from build123d import *

# Parameters (mm, degrees)
SKETCH_2_R          = 21
SKETCH_2_R_2        = 2.5
EXTRUDE_1_DEPTH     = 3
FILLET_1_R          = 1.5
SKETCH_3_R          = 1.45
CUT_EXTRUDE_1_DEPTH = 5
FILLET_2_R          = 3


with BuildPart() as part:
    # Sketch 2 → Extrude 1 (new body)
    with BuildSketch(Plane.XY):
        with BuildLine():
            Line((-10, -58), (10, -58))
            Line((10, -58), (27.296195268, -9.793759437))
            ThreePointArc((27.296195268, -9.793759437), (0, 29), (-27.296195268, -9.793759437))
            Line((-27.296195268, -9.793759437), (-10, -58))
        make_face()
        Circle(SKETCH_2_R, mode=Mode.SUBTRACT)
        with Locations((0, 24.5)):
            Circle(SKETCH_2_R_2, mode=Mode.SUBTRACT)
        with Locations((21.217622393, 12.25)):
            Circle(SKETCH_2_R_2, mode=Mode.SUBTRACT)
        with Locations((21.217622393, -12.25)):
            Circle(SKETCH_2_R_2, mode=Mode.SUBTRACT)
        with Locations((0, -24.5)):
            Circle(SKETCH_2_R_2, mode=Mode.SUBTRACT)
        with Locations((-21.217622393, -12.25)):
            Circle(SKETCH_2_R_2, mode=Mode.SUBTRACT)
        with Locations((-21.217622393, 12.25)):
            Circle(SKETCH_2_R_2, mode=Mode.SUBTRACT)
        with BuildLine():
            Line((-10, -46.155722963), (-10, -27.221315178))
            ThreePointArc((-10, -27.221315178), (-14.496314654, -25.116864085), (-18.567813862, -22.276361651))
            Line((-18.567813862, -22.276361651), (-10, -46.155722963))
        make_face(mode=Mode.SUBTRACT)
        with BuildLine():
            Line((10, -46.155722963), (10, -27.221315178))
            ThreePointArc((10, -27.221315178), (14.496314654, -25.116864085), (18.567813862, -22.276361651))
            Line((18.567813862, -22.276361651), (10, -46.155722963))
        make_face(mode=Mode.SUBTRACT)
    extrude(amount=EXTRUDE_1_DEPTH)

    # Fillet 1
    fillet_1_edges = [part.edges().sort_by_distance(p)[0] for p in [
        (-18.567813862, -22.276361651, 1.5),
        (-10, -46.155722963, 1.5),
        (-10, -27.221315178, 1.5),
        (10, -46.155722963, 1.5),
        (18.567813862, -22.276361651, 1.5),
        (10, -27.221315178, 1.5),
    ]]
    fillet(fillet_1_edges, radius=FILLET_1_R)

    # Sketch 3 → Cut-Extrude 1 (cut)
    with BuildSketch(Plane(origin=(0, 0, 0), x_dir=(-1, 0, 0), z_dir=(0, 0, -1))):
        with Locations((-5, -33)):
            Circle(SKETCH_3_R)
        with Locations((-5, -43)):
            Circle(SKETCH_3_R)
        with Locations((-5, -53)):
            Circle(SKETCH_3_R)
        with Locations((5, -53)):
            Circle(SKETCH_3_R)
        with Locations((5, -43)):
            Circle(SKETCH_3_R)
        with Locations((5, -33)):
            Circle(SKETCH_3_R)
    extrude(amount=-CUT_EXTRUDE_1_DEPTH, mode=Mode.SUBTRACT)

    # Fillet 2
    fillet_2_edges = [part.edges().sort_by_distance(p)[0] for p in [
        (10, -58, 1.5),
        (-10, -58, 1.5),
    ]]
    fillet(fillet_2_edges, radius=FILLET_2_R)


solid = part.part
Read the model definition and answer for the solid it produces. Units are mm, in the model's axes. A direction names the side the tool comes from. Round coordinates to 2 decimals unless told otherwise and drop trailing zeros. Loops run counter-clockwise (first coordinate to the right, second up) from the corner with the lowest first, then second, coordinate; pieces in that order, holes last.
Q1. Section C-C on z = 2.45 is taken. Give the number of separate pieces and of enclosed holes in the cut face, and give its area (3 significant figures).
Q2. Which of the six approach directions +Z, -Z, +X, -X, +Y, -Y give full straight-line access (tool end or side, diameter ignored) to faces 4 (the face through (-11.214, -39.006, 1.521)), 5 (the face through (9.59, -57.47, 1.52))?
Q3. Section B-B on y = 6 is taken. Write down the section's boundary in (x, z), and give its area (3 significant figures).
Q4. Each of these flat-tipped pins is pushed along its axis until it touches: pin 1 (1.5 mm diameter, centred on y = -34, z = 1, fed in from +X); pin 2 (1.5 mm diameter, centred on y = -32, z = 1.5, fed in from -X). Where does it stop, or does it pass through?
Q5. Section D-D on x = 22 is taken. Write down the section's boundary in (y, z), and give its area (3 significant figures).
Q6. Section A-A on x = 0 is taken. Write down the section's boundary in (y, z).
Q7. Determine the mould class of faces 1 (the face through (-21.76, -14.69, 1.48)), 2 (the face through (-4, -21, 3)), 3 (the face through (18.9, -33.2, 1.5)) for opening direction Y: released by +Y, released by -Y, zero draft, split by the parting line, or undercut.
Q8. Consider probe 1 along Y at (x, z) = (5, 1.2); probe 2 along X at (y, z) = (-42.5, 2.55); probe 3 along Y at (x, z) = (-1.5, 0.45). Determine where each line is inside the solid, lowest interval first.
Output:
1. separate pieces: 1
1. enclosed holes: 15
1. area: 2,000 mm2
2. face 4: +Z, -Z
2. face 5: +Z, -Z, +X, -Y
3. outline: (-28.37, 0) - (-20.12, 0) - (-20.12, 3) - (-28.37, 3) - close; (20.12, 0) - (28.37, 0) - (28.37, 3) - (20.12, 3) - close
3. area: 49.5 mm2
4. pin 1: stops at x = 18.88
4. pin 2: stops at x = -19.6
5. outline: (-24.55, 0) - (-14.62, 0) - (-14.62, 3) - (-24.55, 3) - close; (-9.88, 0) - (9.88, 0) - (9.88, 3) - (-9.88, 3) - close; (14.62, 0) - (18.89, 0) - (18.89, 3) - (14.62, 3) - close
5. area: 102 mm2
6. outline: (-58, 0) - (-27, 0) - (-27, 3) - (-58, 3) - close; (-22, 0) - (-21, 0) - (-21, 3) - (-22, 3) - close; (21, 0) - (22, 0) - (22, 3) - (21, 3) - close; (27, 0) - (29, 0) - (29, 3) - (27, 3) - close
7. face 1: undercut
7. face 2: zero draft
7. face 3: released by -Y
8. probe 1: y = -58 to -54.45, -51.55 to -44.45, -41.55 to -34.45, -31.55 to -20.4, 20.4 to 28.57
8. probe 2: x = -15.56 to -6.36, -3.64 to 3.64, 6.36 to 15.56
8. probe 3: y = -58 to -26.5, -22.5 to -20.95, 20.95 to 22.5, 26.5 to 28.96
